Design review of the part built by this model. Coordinates are the model's own, in mm. Round coordinates to 2 decimals unless told otherwise and drop trailing zeros. Loops run counter-clockwise (first coordinate to the right, second up) from the corner with the lowest first, then second, coordinate; pieces in that order, holes last. Notation, with made-up numbers: (-29, 62) -> (11, 62) arc R17 ccw to (11, 68) -> close; hole circle Ø2 at (17, -32). An arc over 180 degrees is marked (long way). Use a Markdown table: item, result. Add a question column.
from build123d import *

# Parameters (mm, degrees)
SKETCH1_R               = 6
BOSS_EXTRUDE1_DEPTH     = 300
SKETCH2_R               = 2.5
CUT_EXTRUDE1_DEPTH      = 20
SKETCH3_R               = 1.5
CUT_EXTRUDE2_DEPTH      = 20
FILLET1_R               = 1
SKETCH4_R               = 1.5
CUT_EXTRUDE3_DEPTH      = 7.0000001
CUT_EXTRUDE3_DEPTH_BACK = 7.000000127


with BuildPart() as part:
    # Sketch1 → Boss-Extrude1 (new body)
    with BuildSketch(Plane(origin=(0, 0, 0), x_dir=(1, 0, 0), z_dir=(0, 1, 0))):
        Circle(SKETCH1_R)
    extrude(amount=BOSS_EXTRUDE1_DEPTH)

    # Sketch2 → Cut-Extrude1 (cut)
    with BuildSketch(Plane.XZ):
        Circle(SKETCH2_R)
    extrude(amount=-CUT_EXTRUDE1_DEPTH, mode=Mode.SUBTRACT)

    # Sketch3 → Cut-Extrude2 (cut)
    with BuildSketch(Plane.XY):
        with Locations((0, 5)):
            Circle(SKETCH3_R)
    extrude(amount=-CUT_EXTRUDE2_DEPTH, mode=Mode.SUBTRACT)

    # Fillet1
    fillet1_edges = [part.edges().sort_by_distance(p)[0] for p in [
        (-6, 0, 0),
        (-6, 300, 0),
    ]]
    fillet(fillet1_edges, radius=FILLET1_R)

    # Sketch4 → Cut-Extrude3 (cut, two sides)
    with BuildSketch(Plane.XY) as cut_extrude3_sk:
        with Locations((0, 225)):
            Circle(SKETCH4_R)
    extrude(amount=CUT_EXTRUDE3_DEPTH, mode=Mode.SUBTRACT)
    extrude(cut_extrude3_sk.sketch, amount=-CUT_EXTRUDE3_DEPTH_BACK, mode=Mode.SUBTRACT)


solid = part.part
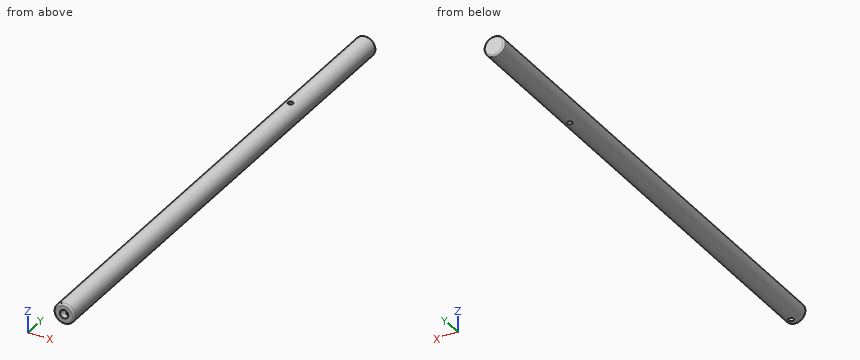
1. Insertion check: P1, Ø4, axis at y = 54.5, z = -3.5, coming from the -X side; P2, Ø1.5, axis at x = -1, y = 77.5, coming from the +Z side; P3, Ø2.5, axis at x = 0, y = 5, coming from the -Z side; P4, Ø6, axis at x = -0.5, y = 229.5, coming from the -Z side. Each pin has a flat end and moves straight along its axis. Give the tip position at first contact, or say it passes through.
2. Consider section A-A on z = 0. State the section outline as (x, y) points.
3. To check wall thickness, follow probe 1 along Y at (x, z) = (0, -4.7); probe 2 along Y at (x, z) = (0, 3.25); probe 3 along Z at (x, y) = (-0.75, 228). State the ranges of each line that lie inside material, in increasing order. Write a range as from..to.
4. Consider section B-B on y = 174.5. State the section outline as (x, z) points.
Verdict:
| question | item | result |
|---|---|---|
| 1 | P1 | stops at x = -5.81 |
| 1 | P2 | stops at z = 5.99 |
| 1 | P3 | stops at z = 2.17 |
| 1 | P4 | stops at z = -6 |
| 2 | outline | (-6, 1) arc R1 ccw to (-5, 0) -> (-2.5, 0) -> (-2.5, 20) -> (2.5, 20) -> (2.5, 0) -> (5, 0) arc R1 ccw to (6, 1) -> (6, 299) arc R1 ccw to (5, 300) -> (-5, 300) arc R1 ccw to (-6, 299) -> close; hole circle Ø3 at (0, 225) |
| 3 | probe 1 | y = 0..3.5, 6.5..223.5, 226.5..300 |
| 3 | probe 2 | y = 0..223.5, 226.5..300 |
| 3 | probe 3 | z = -5.95..5.95 |
| 4 | outline | circle Ø12 at (0, 0) |
